from build123d import *

# Parameters (mm, degrees)
SKETCH_1_R          = 7.5
EXTRUDE_1_DEPTH     = 3
SKETCH_2_R          = 1.75
CUT_EXTRUDE_1_DEPTH = 3


with BuildPart() as part:
    # 草图1 → 凸台-拉伸1 (new body)
    with BuildSketch(Plane.XY):
        Polygon((-14.8, -15), (14.8, -15), (14.8, 0), (27.5, 0), (27.5, 30), (-27.5, 30), (-27.5, 0), (-14.8, 0), align=None)
        with Locations((0, 15)):
            Circle(SKETCH_1_R, mode=Mode.SUBTRACT)
    extrude(amount=EXTRUDE_1_DEPTH)

    # 草图2 → 切除-拉伸1 (cut)
    with BuildSketch(Plane.XY.offset(3)):
        with Locations((-7.5, -7.5)):
            Circle(SKETCH_2_R)
        with Locations(Location((7.5, -7.5, 0), (0, 0, 180))):
            Circle(SKETCH_2_R)
    extrude(amount=-CUT_EXTRUDE_1_DEPTH, mode=Mode.SUBTRACT)


solid = part.part
Build history of the part. All positions in model axes, mm. A direction names the side the tool comes from. Round coordinates to 2 decimals unless told otherwise and drop trailing zeros. Order: outer loops, then holes, each group sorted by start corner. A loop starts at its lowest first (then second) coordinate and runs counter-clockwise, first axis right, second up. Notation, with made-up numbers: M 84,2 L 100,2 A21 cw 100,19 Z; hole C -24.75,-27 d5. An arc over 180 degrees is marked long. Use CSV: the item, a comma, the result in double quotes. Start each with the question number.
(1) Tool access for faces 4 (the face through (0, 30, 1)), 5 (the face through (-21, 0, 1)), 6 (the face through (14.8, -8, 1)): list every direction of +Z, -Z, +X, -X, +Y, -Y with a clear straight run to the whole face (end or side of a thin tool).
(2) Cut at D-D on x = 3. List the corners of the cut face in (y, z).
(3) Flat gauge pins, fed straight in: P1, Ø3, axis at x = -7.5, y = -7.5, coming from the +Z side; P2, Ø1.5, axis at y = -5.5, z = 1.5, coming from the -X side; P3, Ø1.5, axis at x = -21, z = 1, coming from the -Y side. Where does each tip first touch, or does it go through?
(4) Drill centre lines: probe 1 along Y at (x, z) = (0, 1.65); probe 2 along X at (y, z) = (-7, 0.8); probe 3 along Y at (x, z) = (-22.5, 0.8). Where is each one in solid material? Low to high.
(5) Cut at C-C on y = -7.5. List the corners of the cut face in (x, z).
(6) Cut at A-A on y = 21. List the corners of the cut face in (x, z), then the cut area to 3 significant figures.
(7) Cut at B-B on z = 0.45. List the corners of the cut face in (x, y).
(8) Mould opens along Y. For faces 1 (the face through (21, 0, 1)), 2 (the face through (-5.883, -8.17, 1.521)), 3 (the face through (-14.8, -7, 1)) say: +Y half, -Y half, draft (parallel to the pull), parting line (faces both ways), or undercut.
Findings:
1,face 4,"+Z, -Z, +X, -X, +Y"
1,face 5,"+Z, -Z, -X, -Y"
1,face 6,"+Z, -Z, +X, -Y"
2,outline,"M -15,0 L 8.13,0 L 8.13,3 L -15,3 Z; M 21.87,0 L 30,0 L 30,3 L 21.87,3 Z"
3,P1,"passes through"
3,P2,"stops at x = -14.8"
3,P3,"stops at y = 0"
4,probe 1,"y = -15 to 7.5, 22.5 to 30"
4,probe 2,"x = -14.8 to -9.18, -5.82 to 5.82, 9.18 to 14.8"
4,probe 3,"y = 0 to 30"
5,outline,"M -14.8,0 L -9.25,0 L -9.25,3 L -14.8,3 Z; M -5.75,0 L 5.75,0 L 5.75,3 L -5.75,3 Z; M 9.25,0 L 14.8,0 L 14.8,3 L 9.25,3 Z"
6,outline,"M -27.5,0 L -4.5,0 L -4.5,3 L -27.5,3 Z; M 4.5,0 L 27.5,0 L 27.5,3 L 4.5,3 Z"
6,area,"138 mm^2"
7,outline,"M -27.5,0 L -14.8,0 L -14.8,-15 L 14.8,-15 L 14.8,0 L 27.5,0 L 27.5,30 L -27.5,30 Z; hole C -7.5,-7.5 d3.5; hole C 0,15 d15; hole C 7.5,-7.5 d3.5"
8,face 1,"-Y half"
8,face 2,"undercut"
8,face 3,"draft"
